Input: part model. Units: mm. Frame: model coordinates. A direction names the side the tool comes from. Coordinates: 2 decimals unless noted, no trailing zeros. Write each loop counter-clockwise with the first axis right and the second up, starting at its lowest first coordinate (ties: lowest second). Pieces come first, ordered by that corner, then holes. Notation, with made-up numbers: (28, -4) - (76, -4) arc R31 cw to (76, 28) - close; hole circle Ø5 at (39.5, 88.5). An arc over 180 degrees is marked (long way). Use a Markdown table: item, result. Add a question column.
Q1. Pin query (flat end, axial travel): P1, Ø12, axis at x = 37, z = -55, coming from the +Y side; P2, Ø1, axis at x = 19.5, y = 26, coming from the +Z side; P3, Ø17, axis at x = 37.5, z = -13.5, coming from the +Y side. Return the tip coordinate at first contact, or that it passes through.
Q2. Section query B-B (x = 27.5). Return the cut outline in (y, z).
Q3. Material intervals for probe 1 along X at (y, z) = (3, -12); probe 2 along Z at (x, y) = (58, 4); probe 3 along Y at (x, z) = (23, -19.5), sorted ascending. Write a range as from..to.
Q4. Section query D-D (z = -12). Return the cut outline in (x, y).
Q5. Section query A-A (z = -66). Return the cut outline in (x, y), then the cut area to 3 significant figures.
Q6. Mould query, pull axis X, two halves, no side actions, for faces 1 (the face through (35, 27, -41)), 2 (the face through (54, 4, -15)), 3 (the face through (7, 14, -24)). Classes: released by +X, released by -X, zero draft, split by the parting line, or undercut.
Q7. Section query C-C (y = 19). Return the cut outline in (x, z), then the cut area to 3 significant figures.
Q8. Set-up query: faces 4 (the face through (67.48, 34.1, -59.73)), 5 (the face through (40, 31, -34)), 6 (the face through (36.461, 44.646, -63.956)). Return all of +Z, -Z, +X, -X, +Y, -Y with unobstructed straight access to the full face (end or side cutting, diameter ignored); none if empty.
from build123d import *

# Parameters (mm, degrees)
BOSS_EXTRUDE1_DEPTH = 79
SKETCH2_W           = 34
SKETCH2_H           = 36.371997336
CUT_EXTRUDE1_DEPTH  = 71
SKETCH2_4_W         = 34
SKETCH2_4_H         = 36.371997336
CUT_EXTRUDE2_DEPTH  = 79
SKETCH3_W           = 10
SKETCH3_H           = 38
SKETCH3_W_2         = 41.460526603
CUT_EXTRUDE3_DEPTH  = 63.872381388
SKETCH4_W           = 38
SKETCH4_H           = 64.41245134
CUT_EXTRUDE4_DEPTH  = 77.063477679
SKETCH5_R           = 5
CUT_EXTRUDE5_DEPTH  = 8


with BuildPart() as part:
    # Sketch1 → Boss-Extrude1 (new body)
    with BuildSketch(Plane.XY):
        Polygon((78, 33), (0, 69.371997336), (0, 0), (78, 0), align=None)
    extrude(amount=-BOSS_EXTRUDE1_DEPTH)

    # Sketch2 → Cut-Extrude1 (cut)
    with BuildSketch(Plane(origin=(78, 0, 0), x_dir=(0, 0, -1), z_dir=(1, 0, 0))):
        Polygon((0, 33), (0, 7), (34, 32), (34, 33), align=None)
        with Locations((17, 51.185998668)):
            Rectangle(SKETCH2_W, SKETCH2_H)
        Polygon((34, 32), (0, 7), (34, 7), align=None)
    extrude(amount=-CUT_EXTRUDE1_DEPTH, mode=Mode.SUBTRACT)

    # Sketch2<4> → Cut-Extrude2 (cut, through all)
    with BuildSketch(Plane(origin=(78, 0, 0), x_dir=(0, 0, -1), z_dir=(1, 0, 0))):
        with Locations((17, 51.185998668)):
            Rectangle(SKETCH2_4_W, SKETCH2_4_H)
        Polygon((0, 33), (0, 7), (34, 32), (34, 33), align=None)
    extrude(amount=-CUT_EXTRUDE2_DEPTH, mode=Mode.SUBTRACT)

    # Sketch3 → Cut-Extrude3 (cut, through all)
    with BuildSketch(Plane(origin=(26.571016534, 56.981728841, 0), x_dir=(0.906307787, -0.422618262, 0), z_dir=(0.422618262, 0.906307787, 0))):
        with Locations((-24.317872928, 60)):
            Rectangle(SKETCH3_W, SKETCH3_H)
        with Locations((77.475868053, 60)):
            Rectangle(SKETCH3_W_2, SKETCH3_H)
        with Locations((51.745604751, 60)):
            Rectangle(SKETCH3_W, SKETCH3_H)
        with BuildLine():
            ThreePointArc((-3.254395249, 63), (-7.254395249, 59), (-3.254395249, 55))
            Line((-3.254395249, 55), (18.683347003, 55))
            ThreePointArc((18.683347003, 55), (35.745604751, 59), (18.683347003, 63))
            Line((18.683347003, 63), (-3.254395249, 63))
        make_face()
    extrude(amount=-CUT_EXTRUDE3_DEPTH, mode=Mode.SUBTRACT)

    # Sketch4 → Cut-Extrude4 (cut, through all)
    with BuildSketch(Plane(origin=(42.365905596, -19.755546224, 0), x_dir=(0, 0, -1), z_dir=(0.906307787, -0.422618262, 0))):
        with Locations((60, 23.666155718)):
            Rectangle(SKETCH4_W, SKETCH4_H)
    extrude(amount=-CUT_EXTRUDE4_DEPTH, mode=Mode.SUBTRACT)

    # Sketch5 → Cut-Extrude5 (cut, through all)
    with BuildSketch(Plane(origin=(0, 7, 0), x_dir=(1, 0, 0), z_dir=(0, 1, 0))):
        with Locations((20, 12)):
            Circle(SKETCH5_R)
        with Locations((58, 12)):
            Circle(SKETCH5_R)
    extrude(amount=-CUT_EXTRUDE5_DEPTH, mode=Mode.SUBTRACT)


solid = part.part
Values follow:
| question | item | result |
|---|---|---|
| 1 | P1 | y = 54.92 |
| 1 | P2 | z = -34 |
| 1 | P3 | y = 7 |
| 2 | outline | (0, -41) - (48.82, -41) - (48.82, -55) - (56.55, -55) - (56.55, -34) - (7, -34) - (7, 0) - (0, 0) - close; (48.82, -79) - (56.55, -79) - (56.55, -63) - (48.82, -63) - close |
| 3 | probe 1 | 0..15, 25..53, 63..78 |
| 3 | probe 2 | -41..-17, -7..0 |
| 3 | probe 3 | 0..7 |
| 4 | outline | (0, 0) - (15, 0) - (15, 7) - (7, 7) - (7, 15.82) - (0, 15.82) - close; (25, 0) - (53, 0) - (53, 7) - (25, 7) - close; (63, 0) - (78, 0) - (78, 7) - (63, 7) - close |
| 5 | outline | (6.1, 58.8) - (42.73, 41.73) - (45.68, 48.07) - (9.06, 65.15) - close; (52.98, 36.94) - (65.98, 30.88) - (68.94, 37.23) - (55.94, 43.29) - close |
| 5 | area | 383 mm2 |
| 6 | face 1 | zero draft |
| 6 | face 2 | undercut |
| 6 | face 3 | released by +X |
| 7 | outline | (0, -41) - (78, -41) - (78, -34) - (7, -34) - (7, -16.32) - (0, -16.32) - close |
| 7 | area | 670 mm2 |
| 8 | face 4 | -Z, +X, -Y |
| 8 | face 5 | +Z, +X, +Y |
| 8 | face 6 | -Z, -X, -Y |
